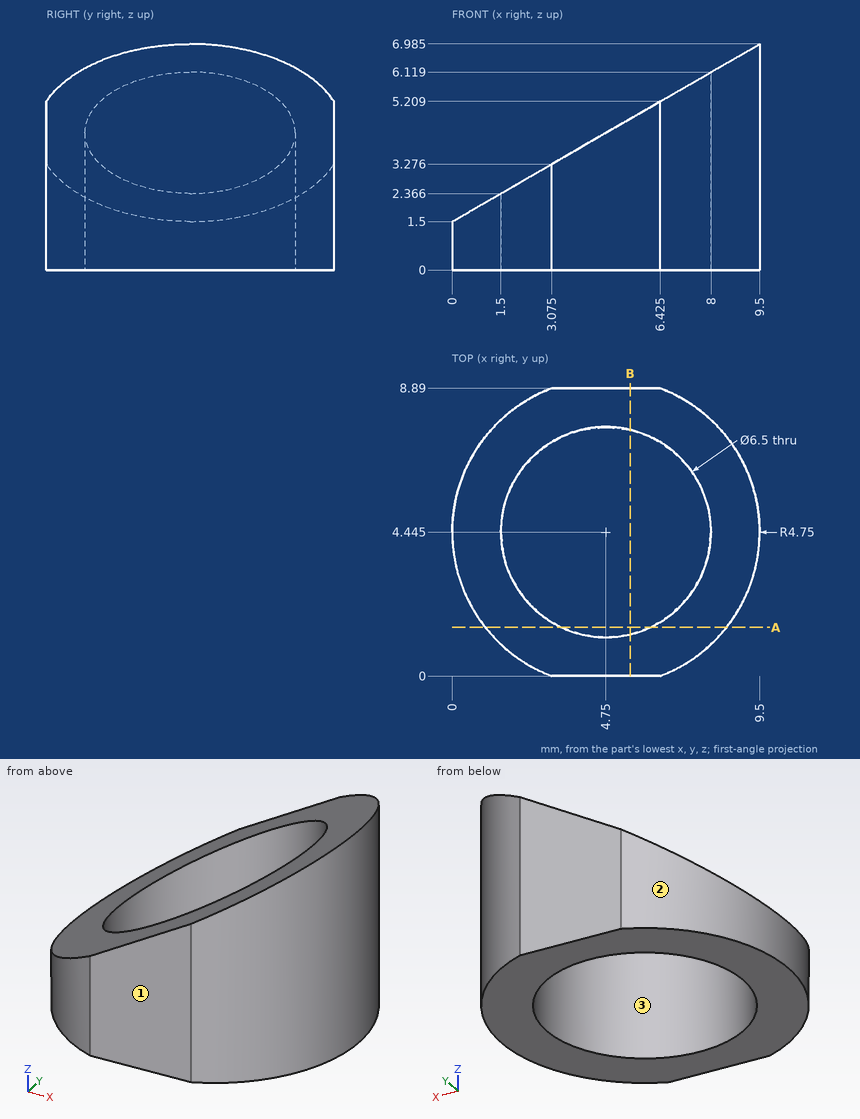
Source: three-view drawing plus pictorial views. Frame: mm from the lowest corner of the part. Give positions to 0.01 mm unless a question says otherwise; leave off trailing zeros. Order: outer loops, then holes, each group sorted by start corner. A loop starts at its lowest first (then second) coordinate and runs counter-clockwise, first axis right, second up. Notation, with made-up numbers: M 80,-2 L 99,-2 A18 ccw 99,17 Z; hole C -11,33 d7. An arc over 180 degrees is marked long. Return JSON: item names as keys, results as strings.
1) Section query A-A on y = 1.5. Output: boundary loops of the cut face in (x, z) (1 decimal).
Taken from the geometry:
{"outline": "M 1,0 L 3.4,0 L 3.4,3.4 L 1,2.1 Z; M 6.1,0 L 8.5,0 L 8.5,6.4 L 6.1,5 Z"}
2) Mould query, pull axis X, two halves, no side actions, for the marked faces 1, 2 and 3. Classes: released by +X, released by -X, zero draft, split by the parting line, or undercut.
Taken from the geometry:
{"face 1": "zero draft", "face 2": "released by -X", "face 3": "undercut"}
3) Line query: L1, parallel to Y at x = 4.75, z = 2.5 (1 decimal); L2, parallel to X at y = 3.25, z = 0.75; L3, parallel to X at y = 5.75, z = 2 (1 decimal). Output: solid intervals per line, ascending. Write a range as [from, to].
Taken from the geometry:
{"L1": "y = [0, 1.2], [7.7, 8.9]", "L2": "x = [0.15, 1.73], [7.77, 9.35]", "L3": "x = [0.9, 1.8], [7.7, 9.3]"}
4) Contact query for a flat-ended pin moving along its axis: pin 1 (1.5 mm diameter, centred on x = 8, z = 5.5, fed in from +Y) (1 decimal). Output: stop coordinate, or through.
Taken from the geometry:
{"pin 1": "stops at y = 8.5"}
5) Section query B-B on x = 5.5. Output: boundary loops of the cut face in (y, z) (1 decimal).
Taken from the geometry:
{"outline": "M 0,0 L 1.3,0 L 1.3,4.7 L 0,4.7 Z; M 7.6,0 L 8.9,0 L 8.9,4.7 L 7.6,4.7 Z"}
